```python
from build123d import *

# Parameters (mm, degrees)
F1_DEPTH = 172.466
F2_W     = 304.8
F2_H     = 177.8
F3_DEPTH = 12.7
F5_R     = 1.75
F6_DEPTH = 15.875
F7_D     = 3.3
F8_D     = 3.3
F9_D     = 24


# Not quite as in the source:
# - a length typed as a fraction of an inch, garbled in the dataset ("3 / 203.2 mm" for 3/8 in), is restored


with BuildPart() as f1:
    # F0 (on Right) → F1 (new body, symmetric)
    with BuildSketch(Plane.YZ):
        with BuildLine():
            Line((-120.2458515259, 50.6342471194), (-135.2673108323, 0))
            Line((-135.2673108323, 0), (-133.7458515259, -0.4513652391))
            Line((-133.7458515259, -0.4513652391), (-119.0612964359, 49.0472471194))
            ThreePointArc((-119.0612964359, 49.0472471194), (-118.4891137925, 49.8676691335), (-117.5398371295, 50.1828818803))
            Line((-117.5398371295, 50.1828818803), (97.0481340778, 50.1828818803))
            ThreePointArc((97.0481340778, 50.1828818803), (97.9974107407, 49.8676691335), (98.5695933841, 49.0472471194))
            Line((98.5695933841, 49.0472471194), (113.2541484741, -0.4513652391))
            Line((113.2541484741, -0.4513652391), (114.7756077805, 0))
            Line((114.7756077805, 0), (99.7541484741, 50.6342471194))
            ThreePointArc((99.7541484741, 50.6342471194), (99.1819658307, 51.4546691335), (98.2326891677, 51.7698818803))
            Line((98.2326891677, 51.7698818803), (-118.7243922195, 51.7698818803))
            ThreePointArc((-118.7243922195, 51.7698818803), (-119.6736688824, 51.4546691335), (-120.2458515259, 50.6342471194))
        make_face()
    extrude(amount=F1_DEPTH, both=True)

    # F2 (on face) → F3 (cut, symmetric)
    with BuildSketch(Plane.XY.offset(51.7698818803)):
        with Locations((0, -10.2458515259)):
            Rectangle(F2_W, F2_H)
    extrude(amount=F3_DEPTH, both=True, mode=Mode.SUBTRACT)

    # F5 (on face) → F6 (join)
    with BuildSketch(Plane(origin=(0, 0, 50.1828818803), x_dir=(1, 0, 0), z_dir=(0, 0, -1))):
        with Locations((132.466, -82.7541484741)):
            Circle(F5_R)
        with Locations((132.466, 103.2458515259)):
            Circle(F5_R)
        with Locations((-132.466, 103.2458515259)):
            Circle(F5_R)
        with Locations((-132.466, -82.7541484741)):
            Circle(F5_R)
    extrude(amount=F6_DEPTH)

    # F7 (through all)
    with Locations(Plane(origin=(0, 105.4912478783, 31.2956660231), x_dir=(-1, 0, 0), z_dir=(0, 0.9587015163, 0.2844141393))):
        with Locations((-9.5, 12)):
            Hole(F7_D / 2)

    # F8 (through all)
    with Locations(Plane(origin=(0, 105.4912478783, 31.2956660231), x_dir=(-1, 0, 0), z_dir=(0, 0.9587015163, 0.2844141393))):
        with Locations((9.5, -12)):
            Hole(F8_D / 2)

    # F9 (through all)
    with Locations(Plane(origin=(0, 105.4912478783, 31.2956660231), x_dir=(-1, 0, 0), z_dir=(0, 0.9587015163, 0.2844141393))):
        with Locations((0, 0)):
            Hole(F9_D / 2)


solid = f1.part
```
Input: part model. Units: mm. Frame: model coordinates. Give positions to 0.01 mm unless a question says otherwise; leave off trailing zeros. Loops run counter-clockwise (first coordinate to the right, second up) from the corner with the lowest first, then second, coordinate; pieces in that order, holes last.
1) Line query: L1, parallel to Y at x = -8, z = 6.5; L2, parallel to Z at x = 18, y = -117; L3, parallel to X at y = 83.5, z = 39. Output: solid intervals per line, ascending.
A:
L1: y = -133.34 to -131.68, 111.19 to 112.85
L2: z = 50.18 to 51.77
L3: x = -134.05 to -130.88, 130.88 to 134.05
2) Section query B-B on x = 83. Return the cut outline in (y, z).
A:
outline: (-135.27, 0) - (-133.75, -0.45) - (-119.06, 49.05) arc R1.59 cw to (-117.54, 50.18) - (-99.15, 50.18) - (-99.15, 51.77) - (-118.72, 51.77) arc R1.59 ccw to (-120.25, 50.63) - close; (78.65, 50.18) - (97.05, 50.18) arc R1.59 cw to (98.57, 49.05) - (113.25, -0.45) - (114.78, 0) - (99.75, 50.63) arc R1.59 ccw to (98.23, 51.77) - (78.65, 51.77) - close
3) Section query A-A on y = 31.5. Return the cut outline in (x, z), and give its area (3 significant figures).
A:
outline: (-172.47, 50.18) - (-152.4, 50.18) - (-152.4, 51.77) - (-172.47, 51.77) - close; (152.4, 50.18) - (172.47, 50.18) - (172.47, 51.77) - (152.4, 51.77) - close
area: 63.7 mm2
4) Section query C-C on x = -0.5. Return the cut outline in (y, z).
A:
outline: (-135.27, 0) - (-133.75, -0.45) - (-119.06, 49.05) arc R1.59 cw to (-117.54, 50.18) - (-99.15, 50.18) - (-99.15, 51.77) - (-118.72, 51.77) arc R1.59 ccw to (-120.25, 50.63) - close; (78.65, 50.18) - (97.05, 50.18) arc R1.59 cw to (98.57, 49.05) - (100.56, 42.34) - (102.08, 42.79) - (99.75, 50.63) arc R1.59 ccw to (98.23, 51.77) - (78.65, 51.77) - close; (107.38, 19.35) - (113.25, -0.45) - (114.78, 0) - (108.9, 19.8) - close
5) Contact query for flat-ended pins moving along their axis: pin 1 (0.5 mm diameter, centred on x = 39.5, z = 51, fed in from +Y); pin 2 (1 mm diameter, centred on x = 132.5, y = 83, fed in from -Z); pin 3 (1.7 mm diameter, centred on x = 33.5, z = 51, fed in from -Y). Output: stop coordinate, or through.
A:
pin 1: stops at y = 99.71
pin 2: stops at z = 34.31
pin 3: stops at y = -120.39
6) Mould query, pull axis Y, two halves, no side actions, for faces 1 (the flat face through (-172.466, -11, 51)), 2 (the flat face through (2.415, -126.506, 23.951)), 3 (the flat face through (2.41, 109.04, 19.34)), 4 (the flat face through (2.41, 107.44, 19.14)). Classes: released by +Y, released by -Y, zero draft, split by the parting line, or undercut.
A:
face 1: zero draft
face 2: undercut
face 3: released by +Y
face 4: undercut
7) Section query D-D on z = 6. Return the cut outline in (x, y), and give its area (3 significant figures).
A:
outline: (-172.47, -133.49) - (172.47, -133.49) - (172.47, -131.83) - (-172.47, -131.83) - close; (-172.47, 111.34) - (172.47, 111.34) - (172.47, 113) - (-172.47, 113) - close
area: 1,140 mm2
